```python
from build123d import *

# Parameters (mm, degrees)
SKETCH1_W      = 80.0862
SKETCH1_H      = 36.0426
EXTRUDE1_DEPTH = 1.524
SKETCH2_W      = 71.3232
SKETCH2_H      = 26.924
EXTRUDE2_DEPTH = 7.747
SKETCH3_R      = 1.397
EXTRUDE3_DEPTH = 45.589607761
SKETCH4_R      = 0.254
EXTRUDE4_DEPTH = 45.589607761


with BuildPart() as part:
    # Sketch1 → Extrude1 (new body)
    with BuildSketch(Plane(origin=(0, 0, 0), x_dir=(1, 0, 0), z_dir=(0, 1, 0))):
        Rectangle(SKETCH1_W, SKETCH1_H)
    extrude(amount=EXTRUDE1_DEPTH)

    # Sketch2 → Extrude2 (add)
    with BuildSketch(Plane(origin=(0, 1.524, 0), x_dir=(1, 0, 0), z_dir=(0, 1, 0))):
        Rectangle(SKETCH2_W, SKETCH2_H)
    extrude(amount=EXTRUDE2_DEPTH)

    # Sketch3 → Extrude3 (cut, through all)
    with BuildSketch(Plane(origin=(0, 1.524, 0), x_dir=(1, 0, 0), z_dir=(0, 1, 0))):
        with Locations(Location((-37.846, 15.875, 0), (0, 0, 270))):
            Circle(SKETCH3_R)
        with Locations(Location((37.846, 15.875, 0), (0, 0, 270))):
            Circle(SKETCH3_R)
        with Locations(Location((37.846, -15.875, 0), (0, 0, 270))):
            Circle(SKETCH3_R)
        with Locations(Location((-37.846, -15.875, 0), (0, 0, 270))):
            Circle(SKETCH3_R)
    extrude(amount=-EXTRUDE3_DEPTH, mode=Mode.SUBTRACT)

    # Sketch4 → Extrude4 (cut, through all)
    with BuildSketch(Plane(origin=(0, 1.524, 0), x_dir=(1, 0, 0), z_dir=(0, 1, 0))):
        with Locations(Location((-34.3281, 15.8877, 0), (0, 0, 270))):
            Circle(SKETCH4_R)
        with Locations(Location((-31.7881, 15.8877, 0), (0, 0, 270))):
            Circle(SKETCH4_R)
        with Locations(Location((-29.2481, 15.8877, 0), (0, 0, 270))):
            Circle(SKETCH4_R)
        with Locations(Location((-26.7081, 15.8877, 0), (0, 0, 270))):
            Circle(SKETCH4_R)
        with Locations(Location((-24.1681, 15.8877, 0), (0, 0, 270))):
            Circle(SKETCH4_R)
        with Locations(Location((-21.6281, 15.8877, 0), (0, 0, 270))):
            Circle(SKETCH4_R)
        with Locations(Location((-19.0881, 15.8877, 0), (0, 0, 270))):
            Circle(SKETCH4_R)
        with Locations(Location((-16.5481, 15.8877, 0), (0, 0, 270))):
            Circle(SKETCH4_R)
        with Locations(Location((-14.0081, 15.8877, 0), (0, 0, 270))):
            Circle(SKETCH4_R)
        with Locations(Location((-11.4681, 15.8877, 0), (0, 0, 270))):
            Circle(SKETCH4_R)
        with Locations(Location((-8.9281, 15.8877, 0), (0, 0, 270))):
            Circle(SKETCH4_R)
        with Locations(Location((-6.3881, 15.8877, 0), (0, 0, 270))):
            Circle(SKETCH4_R)
        with Locations(Location((-3.8481, 15.8877, 0), (0, 0, 270))):
            Circle(SKETCH4_R)
        with Locations(Location((-1.3081, 15.8877, 0), (0, 0, 270))):
            Circle(SKETCH4_R)
        with Locations(Location((1.2319, 15.8877, 0), (0, 0, 270))):
            Circle(SKETCH4_R)
        with Locations(Location((3.7719, 15.8877, 0), (0, 0, 270))):
            Circle(SKETCH4_R)
    extrude(amount=-EXTRUDE4_DEPTH, mode=Mode.SUBTRACT)


solid = part.part
```
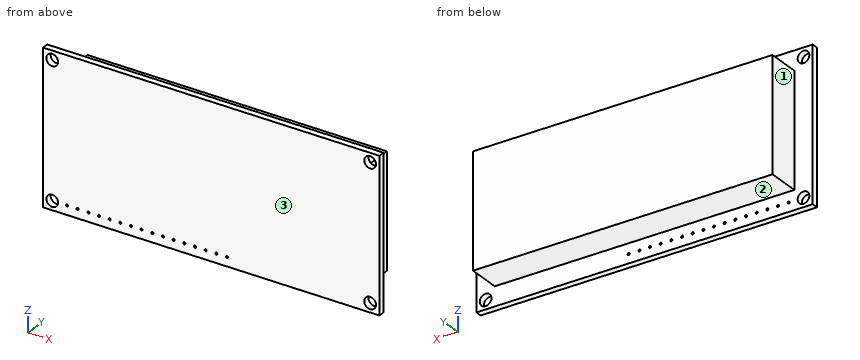
The listing builds one solid part. Answer for the finished solid, in the listing's coordinates (mm). Face numbers are marked on the shaded views. A direction names the side the tool comes from. Give positions to 0.01 mm unless a question says otherwise; leave off trailing zeros. Order: outer loops, then holes, each group sorted by start corner. A loop starts at its lowest first (then second) coordinate and runs counter-clockwise, first axis right, second up.
1) Find section A-A on x = -10. Write down the section's boundary in (y, z).
Reported:
outline: (0, -18.02) - (1.52, -18.02) - (1.52, -13.46) - (9.27, -13.46) - (9.27, 13.46) - (1.52, 13.46) - (1.52, 18.02) - (0, 18.02) - close
2) For the marked faces 1, 2 and 3, determine the directions among +Z, -Z, +X, -X, +Y, -Y from which every point of the face is accessible in a straight line to the end or side of a thin tool.
Reported:
face 1: +Z, -Z, -X, +Y
face 2: -Z, +X, -X, +Y
face 3: +Z, -Z, +X, -X, -Y
3) Find section C-C on y = 8. Write down the section's boundary in (x, z), then the cut area to 3 significant figures.
Reported:
outline: (-35.66, -13.46) - (35.66, -13.46) - (35.66, 13.46) - (-35.66, 13.46) - close
area: 1,920 mm2
4) Consider line 1 along X through (y, z) = (5.5, 10.5); line 2 along Z through (x, y) = (-28, 7.75); line 3 along Y through (x, z) = (27.5, 16.5). Determine where each line is inside the solid, lowest interval first.
Reported:
line 1: x = -35.66 to 35.66
line 2: z = -13.46 to 13.46
line 3: y = 0 to 1.52
5) Given P1, Ø1, axis at y = 3, z = -9, coming from the +X side; P2, Ø4.5, axis at x = 37.846, z = 15.875, coming from the +Y side, each flat-ended and moving along its own axis, determine where each tip first touches the part or whether it passes through.
Reported:
P1: stops at x = 35.66
P2: stops at y = 1.52
6) Find section B-B on z = -6.5. Write down the section's boundary in (x, y), then the cut area to 3 significant figures.
Reported:
outline: (-40.04, 0) - (40.04, 0) - (40.04, 1.52) - (35.66, 1.52) - (35.66, 9.27) - (-35.66, 9.27) - (-35.66, 1.52) - (-40.04, 1.52) - close
area: 675 mm2
